The listing builds one solid part. Answer for the finished solid, in the listing's coordinates (mm). Face numbers are marked on the shaded views. Round coordinates to 2 decimals unless told otherwise and drop trailing zeros. Write each loop counter-clockwise with the first axis right and the second up, starting at its lowest first coordinate (ties: lowest second). Pieces come first, ordered by that corner, then holes. Notation, with made-up numbers: (41.25, 51.5) - (58.25, 51.5) arc R22 cw to (58.25, 62.5) - close; hole circle Ø9 at (23.5, -21). An arc over 180 degrees is marked (long way). Answer as CSV lines item,"result". Start each with the question number.
Item 1: For a pull along Z with two mould halves and no side action, classify the marked faces 1, 2 and 3 as pulls with the +Z half, pulls with the -Z half, needs draft (parallel to the pull), parting line crosses it, or undercut.
Item 2: Straight lines are drawn through the part: line 1 along Z through (x, y) = (13, 210); line 2 along Y through (x, z) = (11.3, 55); line 3 along Z through (x, y) = (20, 165.5). For each, find the intervals that lie inside material, in ascending order. Write a range as [from, to].
Item 3: Flat-ended cylindrical pins translate along their axes: pin 1 (4.5 mm diameter, centred on y = 210, z = -55, fed in from -X); pin 2 (5 mm diameter, centred on y = 177.5, z = -12, fed in from +X); pin 3 (3 mm diameter, centred on x = -4.5, z = -53, fed in from +Y). Find the tip coordinate at first contact, or state that the pin passes through.
Item 4: A cutting plane is placed at A-A on y = 177. Determine the outline of the cut face in (x, z), and give its area (3 significant figures).
```python
from build123d import *

# Parameters (mm, degrees)
BOSS_EXTRUDE1_DEPTH     = 15
BOSS_EXTRUDE3_DEPTH     = 170
SKETCH5_W               = 30
SKETCH5_H               = 10
BOSS_EXTRUDE4_DEPTH     = 30
CIRPATTERN2_COUNT       = 6
CUT_EXTRUDE1_REACH      = 264.726
SKETCH7_W               = 20
SKETCH7_H               = 15
CIRPATTERN4_COUNT       = 6
FILLET1_R               = 5
F_4_0_MM_DOWEL_HOLES1_D = 4
CIRPATTERN8_COUNT       = 6
CUT_EXTRUDE2_REACH      = 257.783
SKETCH11_W              = 30
SKETCH11_H              = 50
M3_CLEARANCE_HOLE1_D    = 3.6
LPATTERN1_COUNT         = 2
LPATTERN1_PITCH         = 31.04
LPATTERN1_COUNT_DIR2    = 2
LPATTERN1_PITCH_DIR2    = 31.04


with BuildPart() as part:
    # Sketch1 → Boss-Extrude1 (new body)
    with BuildSketch(Plane(origin=(0, 0, 0), x_dir=(1, 0, 0), z_dir=(0, 1, 0))):
        Polygon((-69.282032303, 0), (-34.641016151, 60), (34.641016151, 60), (69.282032303, 0), (34.641016151, -60), (-34.641016151, -60), align=None)
    extrude(amount=BOSS_EXTRUDE1_DEPTH)

    # Sketch4 → Boss-Extrude3 (add)
    with BuildSketch(Plane(origin=(0, 15, 0), x_dir=(1, 0, 0), z_dir=(0, 1, 0))):
        Polygon((-34.641016151, -60), (34.641016151, -60), (69.282032303, 0), (57.735026919, 0), (28.867513459, -50), (-28.867513459, -50), (-57.735026919, 0), (-69.282032303, 0), align=None)
    boss_extrude3 = extrude(amount=BOSS_EXTRUDE3_DEPTH)

    # Mirror1: Boss-Extrude3 across plane
    add(boss_extrude3.mirror(Plane(origin=(57.735026919, 185, 0), x_dir=(1, 0, 0), z_dir=(0, 0, 1))))

    # Sketch5 → Boss-Extrude4 (add)
    with BuildSketch(Plane(origin=(0, 185, 0), x_dir=(1, 0, 0), z_dir=(0, 1, 0))):
        with Locations((0, -55)):
            Rectangle(SKETCH5_W, SKETCH5_H)
    boss_extrude4 = extrude(amount=BOSS_EXTRUDE4_DEPTH)

    # CirPattern2: Boss-Extrude4 ×6 about axis
    cirpattern2_axis = Axis((0, 0, 0), (0, 1, 0))
    for i in range(1, CIRPATTERN2_COUNT):
        add(boss_extrude4.rotate(cirpattern2_axis, i * 360 / CIRPATTERN2_COUNT))

    # Sketch7 → Cut-Extrude1 (cut, up to next)
    with BuildSketch(Plane(origin=(-51.961524227, 0, 30), x_dir=(0.49999999999999695, 0, 0.8660254037844404), z_dir=(-0.8660254037844404, 0, 0.49999999999999695)), mode=Mode.PRIVATE) as cut_extrude1_sk1:
        with Locations((0, 207.5)):
            Rectangle(SKETCH7_W, SKETCH7_H)
    cut_extrude1_tool1 = extrude(cut_extrude1_sk1.sketch, amount=-CUT_EXTRUDE1_REACH, mode=Mode.PRIVATE) & part.part
    cut_extrude1 = cut_extrude1_tool1.solids().sort_by_distance((-51.961524, 207.5, 30))[0]
    add(cut_extrude1, mode=Mode.SUBTRACT)

    # CirPattern4: Cut-Extrude1 ×6 about axis
    cirpattern4_axis = Axis((0, 0, 0), (0, 1, 0))
    for i in range(1, CIRPATTERN4_COUNT):
        add(cut_extrude1.rotate(cirpattern4_axis, i * 360 / CIRPATTERN4_COUNT), mode=Mode.SUBTRACT)

    # Fillet1
    fillet1_edges = [part.edges().sort_by_distance(p)[0] for p in [
        (-55.131397208, 185, 14.509618943),
        (-40.131397208, 185, 40.490381057),
        (-40.131397208, 185, -40.490381057),
        (-55.131397208, 185, -14.509618943),
        (15, 185, -55),
        (-15, 185, -55),
        (55.131397208, 185, -14.509618943),
        (40.131397208, 185, -40.490381057),
        (40.131397208, 185, 40.490381057),
        (55.131397208, 185, 14.509618943),
        (-15, 185, 55),
        (15, 185, 55),
    ]]
    fillet(fillet1_edges, radius=FILLET1_R)
    fillet1_2_edges = [part.edges().sort_by_distance(p)[0] for p in [
        (-49.551270189, 215, 14.174682453),
        (-58.211524227, 215, 19.174682453),
        (-37.051270189, 215, -35.825317547),
        (-45.711524227, 215, -40.825317547),
        (12.5, 215, -50),
        (12.5, 215, -60),
        (49.551270189, 215, -14.174682453),
        (58.211524227, 215, -19.174682453),
        (37.051270189, 215, 35.825317547),
        (45.711524227, 215, 40.825317547),
        (-37.051270189, 215, 35.825317547),
        (-45.711524227, 215, 40.825317547),
        (49.551270189, 215, 14.174682453),
        (58.211524227, 215, 19.174682453),
        (-49.551270189, 215, -14.174682453),
        (-58.211524227, 215, -19.174682453),
        (-12.5, 215, -50),
        (-12.5, 215, -60),
        (37.051270189, 215, -35.825317547),
        (45.711524227, 215, -40.825317547),
        (12.5, 215, 50),
        (12.5, 215, 60),
        (-12.5, 215, 50),
        (-12.5, 215, 60),
    ]]
    fillet(fillet1_2_edges, radius=FILLET1_R - 0.0001)  # a hair under: the kernel refuses the full size

    # Ø4.0 mm Dowel Holes1 (through all)
    with Locations(Plane(origin=(15, 0, 0), x_dir=(0, 0, -1), z_dir=(1, 0, 0))):
        with Locations((-55, 210)):
            f_4_0_mm_dowel_holes1 = Hole(F_4_0_MM_DOWEL_HOLES1_D / 2)

    # CirPattern8: Ø4.0 mm Dowel Holes1 ×6 about axis
    cirpattern8_axis = Axis((0, 15, 0), (0, -1, 0))
    for i in range(1, CIRPATTERN8_COUNT):
        add(f_4_0_mm_dowel_holes1.rotate(cirpattern8_axis, i * 360 / CIRPATTERN8_COUNT), mode=Mode.SUBTRACT)

    # Sketch11 → Cut-Extrude2 (cut, up to next)
    with BuildSketch(Plane.XY.offset(60), mode=Mode.PRIVATE) as cut_extrude2_sk1:
        with Locations((0, 40)):
            Rectangle(SKETCH11_W, SKETCH11_H)
    cut_extrude2_tool1 = extrude(cut_extrude2_sk1.sketch, amount=-CUT_EXTRUDE2_REACH, mode=Mode.PRIVATE) & part.part
    add(cut_extrude2_tool1.solids().sort_by_distance((0, 40, 60))[0], mode=Mode.SUBTRACT)

    # M3 Clearance Hole1 (through all)
    with Locations(Plane(origin=(0, 0, 0), x_dir=(-1, 0, 0), z_dir=(0, -1, 0))):
        with Locations((-15.52, 15.52)):
            m3_clearance_hole1 = Hole(M3_CLEARANCE_HOLE1_D / 2)

    # LPattern1: M3 Clearance Hole1 2 × 2
    with Locations(*[(-i * LPATTERN1_PITCH, 0, j * LPATTERN1_PITCH_DIR2) for i in range(LPATTERN1_COUNT) for j in range(LPATTERN1_COUNT_DIR2) if (i, j) != (0, 0)]):
        add(m3_clearance_hole1, mode=Mode.SUBTRACT)


solid = part.part
```
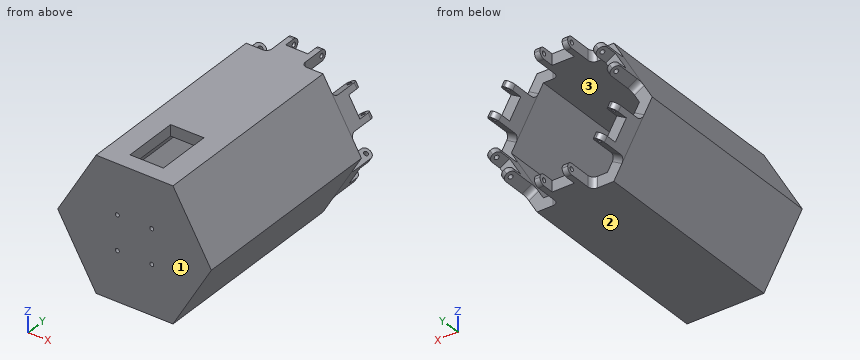
Geometry says:
1,face 1,"needs draft"
1,face 2,"pulls with the -Z half"
1,face 3,"undercut"
2,line 1,"z = [-60, -57], [-53, -50], [50, 53], [57, 60]"
2,line 2,"y = [0, 15], [65, 208], [212, 215]"
2,line 3,"z = [-60, -50], [50, 60]"
3,pin 1,"stops at x = -15"
3,pin 2,"stops at x = 63.8"
3,pin 3,"stops at y = 200"
4,outline,"(-69.28, 0) - (-34.64, -60) - (34.64, -60) - (69.28, 0) - (34.64, 60) - (-34.64, 60) - close; hole (-57.74, 0) - (-28.87, -50) - (28.87, -50) - (57.74, 0) - (28.87, 50) - (-28.87, 50) - close"
4,area,"3,810 mm^2"
